Read the model definition and answer for the solid it produces. Units are mm, in the model's axes. A direction names the side the tool comes from. Give positions to 0.01 mm unless a question says otherwise; leave off trailing zeros. Order: outer loops, then holes, each group sorted by start corner. A loop starts at its lowest first (then second) coordinate and runs counter-clockwise, first axis right, second up. Notation, with made-up numbers: (-2.5, 34) - (5.5, 34) arc R21 ccw to (5.5, 43) - close; hole circle Ø8 at (28.5, 71). An arc over 180 degrees is marked (long way). Write each question's results on one line, items separated by ' | '.
from build123d import *

# Parameters (mm, degrees)
SKETCH1_R           = 3.175
BOSS_EXTRUDE1_DEPTH = 6.604
SKETCH2_R           = 2.38125
BOSS_EXTRUDE2_DEPTH = 3.175
SKETCH2_3_R         = 2.38125
BOSS_EXTRUDE3_DEPTH = 9.525
SKETCH4_R           = 3.81
BOSS_EXTRUDE4_DEPTH = 3.175
BOSS_EXTRUDE5_START = 3.175
BOSS_EXTRUDE5_DEPTH = 3.175


with BuildPart() as part:
    # Sketch1 → Boss-Extrude1 (new body)
    with BuildSketch(Plane(origin=(0, 0, 0), x_dir=(1, 0, 0), z_dir=(0, 1, 0))):
        with Locations(Location((0, 0, 0), (0, 0, 90))):
            Circle(SKETCH1_R)
    extrude(amount=BOSS_EXTRUDE1_DEPTH)

    # Sketch2 → Boss-Extrude2 (add)
    with BuildSketch(Plane(origin=(0, 6.604, 0), x_dir=(1, 0, 0), z_dir=(0, 1, 0))):
        with BuildLine():
            Line((0, -3.81), (-12.7, -3.81))
            ThreePointArc((-12.7, -3.81), (-16.51, 0), (-12.7, 3.81))
            Line((-12.7, 3.81), (0, 3.81))
            ThreePointArc((0, 3.81), (3.81, 0), (0, -3.81))
        make_face()
        with Locations(Location((-12.7, 0, 0), (0, 0, 270))):
            Circle(SKETCH2_R, mode=Mode.SUBTRACT)
    extrude(amount=BOSS_EXTRUDE2_DEPTH)

    # Sketch2_3 → Boss-Extrude3 (add)
    with BuildSketch(Plane(origin=(0, 6.604, 0), x_dir=(1, 0, 0), z_dir=(0, 1, 0))):
        with Locations(Location((-12.7, 0, 0), (0, 0, 90))):
            Circle(SKETCH2_3_R)
    extrude(amount=BOSS_EXTRUDE3_DEPTH)

    # Sketch4 → Boss-Extrude4 (add)
    with BuildSketch(Plane(origin=(0, 16.129, 0), x_dir=(1, 0, 0), z_dir=(0, 1, 0))):
        with Locations(Location((-12.7, 0, 0), (0, 0, 270))):
            Circle(SKETCH4_R)
    extrude(amount=BOSS_EXTRUDE4_DEPTH)

    # Sketch5 → Boss-Extrude5 (add)
    with BuildSketch(Plane.XZ.offset(BOSS_EXTRUDE5_START)):
        with BuildLine():
            Line((0.986100562, 3.680177398), (19.386987553, -1.250325411))
            ThreePointArc((19.386987553, -1.250325411), (22.081064389, -5.916603371), (17.414786429, -8.610680207))
            Line((17.414786429, -8.610680207), (-0.986100562, -3.680177398))
            ThreePointArc((-0.986100562, -3.680177398), (-3.680177398, 0.986100562), (0.986100562, 3.680177398))
        make_face()
    extrude(amount=-BOSS_EXTRUDE5_DEPTH)


solid = part.part
(1) Section D-D (x = 19) is taken. Give the vertices of the cut face in (y, z) (3 decimals).
Conclusion:
outline: (-3.175, -8.693) - (0, -8.693) - (0, -1.147) - (-3.175, -1.147) - close
(2) Section A-A (x = -9.5) is taken. Give the vertices of the cut face in (y, z), plus the area to 3 significant figures.
Conclusion:
outline: (6.6, -3.81) - (9.78, -3.81) - (9.78, 3.81) - (6.6, 3.81) - close; (16.13, -2.07) - (19.3, -2.07) - (19.3, 2.07) - (16.13, 2.07) - close | area: 37.3 mm^2
(3) Section C-C (y = 12) is taken. Give the vertices of the cut face in (x, z).
Conclusion:
outline: circle Ø4.76 at (-12.7, 0)
(4) The mould has two halves that part along Y. Classify faces 1 (the face through (9, -3.175, -2)), 2 (the face through (-3.701, -1.61, 0.905)), 3 (the face through (-15.06, 12.91, 0.31)): pulls with the +Y half, pulls with the -Y half, needs draft (parallel to the pull), parting line crosses it, or undercut.
Conclusion:
face 1: pulls with the -Y half | face 2: needs draft | face 3: undercut
(5) Consider probe 1 along Y at (x, z) = (-13.5, -3.5); probe 2 along Y at (x, z) = (8, -5.25) (3 decimals); probe 3 along Y at (x, z) = (-12.5, 0). Determine where each line is inside the solid, lowest interval first. Write a range as [from, to].
Conclusion:
probe 1: [6.6, 9.78], [16.13, 19.3] | probe 2: [-3.175, 0] | probe 3: [6.6, 19.3]
(6) For faces 4 (the face through (-16.51, 8.17, 0.08)), 5 (the face through (1.93, 3.26, 2.52)), 6 (the face through (-6, 8, 3.81)), 7 (the face through (-16.42, 17.69, -0.83)), 8 (the face through (3.81, 8.17, -0.08)), determine the directions among +Z, -Z, +X, -X, +Y, -Y from which every point of the face is accessible in a straight line to the end or side of a thin tool.
Conclusion:
face 4: -X, +Y, -Y | face 5: none | face 6: +Z, +X, -X, +Y, -Y | face 7: +Y | face 8: +X, +Y
(7) Each of these flat-tipped pins is pushed along its axis until it touches: pin 1 (6.5 mm diameter, centred on x = 7, z = -3.5, fed in from +Y); pin 2 (1 mm diameter, centred on x = 0.5, z = 0, fed in from +Y); pin 3 (6 mm diameter, centred on x = -11.5, z = 1.5, fed in from -Y). Where does it stop, or does it pass through?
Conclusion:
pin 1: y = 0 | pin 2: y = 9.78 | pin 3: y = 6.6
(8) Section B-B (z = 0) is taken. Give the vertices of the cut face in (x, y) (3 decimals).
Conclusion:
outline: (-16.51, 6.604) - (-3.175, 6.604) - (-3.175, 0) - (-3.81, 0) - (-3.81, -3.175) - (14.721, -3.175) - (14.721, 0) - (3.175, 0) - (3.175, 6.604) - (3.81, 6.604) - (3.81, 9.779) - (-10.319, 9.779) - (-10.319, 16.129) - (-8.89, 16.129) - (-8.89, 19.304) - (-16.51, 19.304) - (-16.51, 16.129) - (-15.081, 16.129) - (-15.081, 9.779) - (-16.51, 9.779) - close
